Source: CAD feature listing. Evaluate the final solid. Frame: model axes, mm. A direction names the side the tool comes from. Coordinates: 2 decimals unless noted, no trailing zeros. Order: outer loops, then holes, each group sorted by start corner. A loop starts at its lowest first (then second) coordinate and runs counter-clockwise, first axis right, second up.
```python
from build123d import *

# Parameters (mm, degrees)
SKETCH1_R                      = 6.05
SKETCH1_R_2                    = 3.05
BOSS_EXTRUDE1_DEPTH            = 10
SKETCH2_R                      = 17.5
BOSS_EXTRUDE2_DEPTH            = 6.5
CUT_EXTRUDE1_REACH             = 28.693
SKETCH3_R                      = 1.25
CUT_EXTRUDE2_DEPTH             = 30.744747435
CUT_EXTRUDE2_DEPTH_BACK        = 30.744747435
SKETCH4_R                      = 1.5
CUT_EXTRUDE3_REACH             = 28.693
SKETCH6_R                      = 3.2
CUT_EXTRUDE3_DIRECTION_2_REACH = 28.693
BOSS_EXTRUDE3_DEPTH            = 16.5
SKETCH8_W                      = 5.75
SKETCH8_H                      = 2.75
CUT_EXTRUDE4_DEPTH             = 5
CUT_EXTRUDE5_DEPTH             = 2.75
CIRPATTERN1_START              = 11.875
CIRPATTERN1_OUTLINE_R          = 1.25
CIRPATTERN1_DEPTH              = 2.75


# Read off the part's stored shape, not the designer's step: CirPattern1
with BuildPart() as part:
    # Sketch1 → Boss-Extrude1 (new body)
    with BuildSketch(Plane(origin=(0, 0, 0), x_dir=(1, 0, 0), z_dir=(0, 1, 0))):
        with Locations(Location((0, 0, 0), (0, 0, 270))):
            Circle(SKETCH1_R)
        with Locations(Location((0, 0, 0), (0, 0, 270))):
            Circle(SKETCH1_R_2, mode=Mode.SUBTRACT)
    extrude(amount=BOSS_EXTRUDE1_DEPTH)

    # Sketch2 → Boss-Extrude2 (add)
    with BuildSketch(Plane(origin=(0, 10, 0), x_dir=(1, 0, 0), z_dir=(0, 1, 0))):
        with Locations(Location((0, 0, 0), (0, 0, 90))):
            Circle(SKETCH2_R)
    extrude(amount=BOSS_EXTRUDE2_DEPTH)

    # Sketch3 → Cut-Extrude1 (cut, up to next)
    with BuildSketch(Plane.XZ.offset(-10), mode=Mode.PRIVATE) as cut_extrude1_sk1:
        with Locations(Location((12.1, 0, 0), (0, 0, 270))):
            Circle(SKETCH3_R)
    cut_extrude1_tool1 = extrude(cut_extrude1_sk1.sketch, amount=-CUT_EXTRUDE1_REACH, mode=Mode.PRIVATE) & part.part
    # Sketch3 → Cut-Extrude1 (cut, up to next)
    with BuildSketch(Plane.XZ.offset(-10), mode=Mode.PRIVATE) as cut_extrude1_sk2:
        with Locations(Location((0, -12.1, 0), (0, 0, 270))):
            Circle(SKETCH3_R)
    cut_extrude1_tool2 = extrude(cut_extrude1_sk2.sketch, amount=-CUT_EXTRUDE1_REACH, mode=Mode.PRIVATE) & part.part
    # Sketch3 → Cut-Extrude1 (cut, up to next)
    with BuildSketch(Plane.XZ.offset(-10), mode=Mode.PRIVATE) as cut_extrude1_sk3:
        with Locations(Location((-12.1, 0, 0), (0, 0, 270))):
            Circle(SKETCH3_R)
    cut_extrude1_tool3 = extrude(cut_extrude1_sk3.sketch, amount=-CUT_EXTRUDE1_REACH, mode=Mode.PRIVATE) & part.part
    # Sketch3 → Cut-Extrude1 (cut, up to next)
    with BuildSketch(Plane.XZ.offset(-10), mode=Mode.PRIVATE) as cut_extrude1_sk4:
        with Locations(Location((0, 12.1, 0), (0, 0, 270))):
            Circle(SKETCH3_R)
    cut_extrude1_tool4 = extrude(cut_extrude1_sk4.sketch, amount=-CUT_EXTRUDE1_REACH, mode=Mode.PRIVATE) & part.part
    add(cut_extrude1_tool1.solids().sort_by_distance((12.1, 10, 0))[0], mode=Mode.SUBTRACT)
    add(cut_extrude1_tool2.solids().sort_by_distance((0, 10, -12.1))[0], mode=Mode.SUBTRACT)
    add(cut_extrude1_tool3.solids().sort_by_distance((-12.1, 10, 0))[0], mode=Mode.SUBTRACT)
    add(cut_extrude1_tool4.solids().sort_by_distance((0, 10, 12.1))[0], mode=Mode.SUBTRACT)

    # Sketch4 → Cut-Extrude2 (cut, two sides: drawn at the far end of the back side and taken through both)
    with BuildSketch(Plane.XY.offset(-CUT_EXTRUDE2_DEPTH_BACK)):
        with Locations((0, 4.916404418)):
            Circle(SKETCH4_R)
    extrude(amount=CUT_EXTRUDE2_DEPTH + CUT_EXTRUDE2_DEPTH_BACK, mode=Mode.SUBTRACT)

    # Sketch6 → Cut-Extrude3 (cut, up to next)
    with BuildSketch(Plane(origin=(0, 10, 0), x_dir=(-1, 0, 0), z_dir=(0, -1, 0)), mode=Mode.PRIVATE) as cut_extrude3_sk1:
        with Locations(Location((0, 0, 0), (0, 0, 270))):
            Circle(SKETCH6_R)
    cut_extrude3_tool1 = extrude(cut_extrude3_sk1.sketch, amount=-CUT_EXTRUDE3_REACH, mode=Mode.PRIVATE) & part.part
    add(cut_extrude3_tool1.solids().sort_by_distance((0, 10, 0))[0], mode=Mode.SUBTRACT)

    # Sketch6 → Cut-Extrude3 direction 2 (cut, up to next)
    with BuildSketch(Plane(origin=(0, 10, 0), x_dir=(-1, 0, 0), z_dir=(0, -1, 0)), mode=Mode.PRIVATE) as cut_extrude3_direction_2_sk1:
        with Locations(Location((0, 0, 0), (0, 0, 270))):
            Circle(SKETCH6_R)
    cut_extrude3_direction_2_tool1 = extrude(cut_extrude3_direction_2_sk1.sketch, amount=CUT_EXTRUDE3_DIRECTION_2_REACH, mode=Mode.PRIVATE) & part.part
    add(cut_extrude3_direction_2_tool1.solids().sort_by_distance((0, 10, 0))[0], mode=Mode.SUBTRACT)

    # Sketch7 → Boss-Extrude3 (add)
    with BuildSketch(Plane.XZ):
        with BuildLine():
            Line((-1.717556404, 2.7), (1.717556404, 2.7))
            ThreePointArc((1.717556404, 2.7), (0, 3.2), (-1.717556404, 2.7))
        make_face()
    extrude(amount=-BOSS_EXTRUDE3_DEPTH)

    # Sketch8 → Cut-Extrude4 (cut)
    with BuildSketch(Plane(origin=(17.5, 0, 0), x_dir=(0, 0, -1), z_dir=(1, 0, 0))):
        with Locations((0, 13.25)):
            Rectangle(SKETCH8_W, SKETCH8_H)
    extrude(amount=-CUT_EXTRUDE4_DEPTH, mode=Mode.SUBTRACT)

    # Sketch9 → Cut-Extrude5 (cut)
    with BuildSketch(Plane.XZ.offset(-14.625)):
        Polygon((15.419764048, 0), (13.759882024, 2.875), (10.440117976, 2.875), (8.780235952, 0), (10.440117976, -2.875), (13.759882024, -2.875), align=None)
    extrude(amount=CUT_EXTRUDE5_DEPTH, mode=Mode.SUBTRACT)

    # CirPattern1 outline → CirPattern1 (cut)
    # profile 1 of 3: a face of its own
    with BuildSketch(Plane(origin=(0, 0, 0), x_dir=(1, 0, 0), z_dir=(0, 1, 0)).offset(CIRPATTERN1_START)):
        with BuildLine():
            Line((-8.780235952, 0), (-10.440117976, 2.875))
            Line((-10.440117976, 2.875), (-17.26222393, 2.875))
            ThreePointArc((-17.26222393, 2.875), (-17.5, 0), (-17.26222393, -2.875))
            Line((-17.26222393, -2.875), (-10.440117976, -2.875))
            Line((-10.440117976, -2.875), (-8.780235952, 0))
        make_face()
        with Locations((-12.1, 0)):
            Circle(CIRPATTERN1_OUTLINE_R, mode=Mode.SUBTRACT)
    # profile 2 of 3: a face of its own
    with BuildSketch(Plane(origin=(0, 0, 0), x_dir=(1, 0, 0), z_dir=(0, 1, 0)).offset(CIRPATTERN1_START)):
        with BuildLine():
            ThreePointArc((2.875, 17.26222393), (0, 17.5), (-2.875, 17.26222393))
            Line((-2.875, 17.26222393), (-2.875, 10.440117976))
            Line((-2.875, 10.440117976), (0, 8.780235952))
            Line((0, 8.780235952), (2.875, 10.440117976))
            Line((2.875, 10.440117976), (2.875, 17.26222393))
        make_face()
        with Locations((0, 12.1)):
            Circle(CIRPATTERN1_OUTLINE_R, mode=Mode.SUBTRACT)
    # profile 3 of 3: a face of its own
    with BuildSketch(Plane(origin=(0, 0, 0), x_dir=(1, 0, 0), z_dir=(0, 1, 0)).offset(CIRPATTERN1_START)):
        with BuildLine():
            Line((-2.875, -10.440117976), (-2.875, -17.26222393))
            ThreePointArc((-2.875, -17.26222393), (0, -17.5), (2.875, -17.26222393))
            Line((2.875, -17.26222393), (2.875, -10.440117976))
            Line((2.875, -10.440117976), (0, -8.780235952))
            Line((0, -8.780235952), (-2.875, -10.440117976))
        make_face()
        with Locations((0, -12.1)):
            Circle(CIRPATTERN1_OUTLINE_R, mode=Mode.SUBTRACT)
    extrude(amount=CIRPATTERN1_DEPTH, mode=Mode.SUBTRACT)


solid = part.part
```
1. Draft query along Z for faces 5 (the face through (1.82, 4.93, 5.77)), 6 (the face through (2.875, 13, -14)), 7 (the face through (14, 14.625, 0)), 8 (the face through (0.38, 15.55, 10.91)). Return one class per face: released by +Z, released by -Z, zero draft, split by the parting line, or undercut.
Findings:
face 5: split by the parting line
face 6: zero draft
face 7: undercut
face 8: undercut
2. Ray query, line 1 (Y direction, x = 2, z = 12) (3 decimals); line 2 (X direction, y = 15.3, z = 0); line 3 (Y direction, x = 4, z = -8). Return the intervals inside material, ascending.
Findings:
line 1: y = 10 to 11.875, 14.625 to 16.5
line 2: x = -17.5 to -13.35, -10.85 to -3.2, 3.2 to 10.85, 13.35 to 17.5
line 3: y = 10 to 16.5
3. Access query for faces 1 (the face through (-2.875, 13, 14)), 2 (the face through (-14, 11.875, 0)), 3 (the face through (-2.875, 13, -14)), 4 (the face through (-0.1, 8.1, -3.2)). Directions: +Z, -Z, +X, -X, +Y, -Y. A direction counts if a zero-diameter tool reaches every point of the face in a straight line with its end or side. Return the directions, or none.
Findings:
face 1: +Z
face 2: -X
face 3: -Z
face 4: +Y, -Y
4. Section query C-C on x = 12.1. Return loops of the section in (y, z) (3 decimals).
Findings:
outline: (10, -12.643) - (16.5, -12.643) - (16.5, -1.25) - (14.625, -1.25) - (14.625, -2.875) - (11.875, -2.875) - (11.875, -1.25) - (10, -1.25) - close; (10, 1.25) - (11.875, 1.25) - (11.875, 2.875) - (14.625, 2.875) - (14.625, 1.25) - (16.5, 1.25) - (16.5, 12.643) - (10, 12.643) - close
5. Section query A-A on y = 10.75. Return loops of the section in (x, z).
Findings:
outline: circle Ø35 at (0, 0); hole circle Ø2.5 at (-12.1, 0); hole (-1.72, 2.7) arc R3.2 ccw (long way) to (1.72, 2.7) - close; hole circle Ø2.5 at (0, -12.1); hole circle Ø2.5 at (0, 12.1); hole circle Ø2.5 at (12.1, 0)
6. Section query B-B on z = -12.1. Return loops of the section in (x, y) (3 decimals).
Findings:
outline: (-12.643, 10) - (-1.25, 10) - (-1.25, 11.875) - (-2.875, 11.875) - (-2.875, 14.625) - (-1.25, 14.625) - (-1.25, 16.5) - (-12.643, 16.5) - close; (1.25, 10) - (12.643, 10) - (12.643, 16.5) - (1.25, 16.5) - (1.25, 14.625) - (2.875, 14.625) - (2.875, 11.875) - (1.25, 11.875) - close
7. Section query D-D on x = -10. Return loops of the section in (y, z) (3 decimals), plus the area to 3 significant figures.
Findings:
outline: (10, -14.361) - (16.5, -14.361) - (16.5, 14.361) - (10, 14.361) - close; hole (11.875, -2.113) - (14.625, -2.113) - (14.625, 2.113) - (11.875, 2.113) - close
area: 175 mm2
8. Pin query (flat end, axial travel): P1, Ø12, axis at x = 2.5, z = 12, coming from the -Y side; P2, Ø2, axis at x = -12.5, y = 13.5, coming from the -Z side; P3, Ø2, axis at x = 15, y = 12.5, coming from the -Z side; P4, Ø10.5, axis at x = -2, z = 5, coming from the -Y side. Return the tip coordinate at first contact, or that it passes through.
Findings:
P1: stops at y = 10
P2: stops at z = -13.19
P3: stops at z = -10.5
P4: stops at y = 0
